Build history of the part. All positions in model axes, mm. Face numbers are marked on the shaded views. Round coordinates to 2 decimals unless told otherwise and drop trailing zeros. Order: outer loops, then holes, each group sorted by start corner. A loop starts at its lowest first (then second) coordinate and runs counter-clockwise, first axis right, second up. Notation, with made-up numbers: M -19.75,-11.75 L 19.25,-11.75 A13 cw 19.25,-7.75 Z; hole C -21.75,17.25 d4. An arc over 180 degrees is marked long. Use CSV: the item, a comma, the result in double quotes.
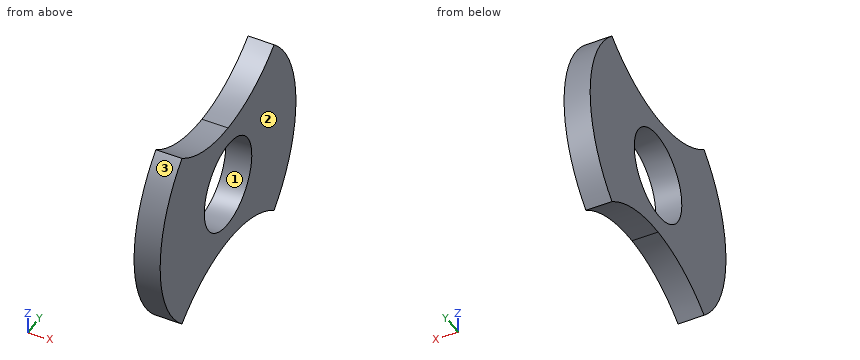
from build123d import *

# Parameters (mm, degrees)
BOSS_EXTRUDE1_DEPTH = 10
SKETCH3_R           = 17.5
CUT_EXTRUDE3_DEPTH  = 63.842489918


with BuildPart() as part:
    # Sketch1 → Boss-Extrude1 (new body)
    with BuildSketch(Plane(origin=(0, 0, 0), x_dir=(0, 0, -1), z_dir=(1, 0, 0))):
        with BuildLine():
            ThreePointArc((-36.722656494, 33.942179351), (-28.013204115, 17.954750168), (-25, 0))
            ThreePointArc((-25, 0), (-28.013204115, -17.954750168), (-36.722656494, -33.942179351))
            ThreePointArc((-36.722656494, -33.942179351), (0, -50.00625), (36.722656494, -33.942179351))
            ThreePointArc((36.722656494, -33.942179351), (28.013204115, -17.954750168), (25, 0))
            ThreePointArc((25, 0), (28.013204115, 17.954750168), (36.722656494, 33.942179351))
            ThreePointArc((36.722656494, 33.942179351), (0, 50.00625), (-36.722656494, 33.942179351))
        make_face()
    extrude(amount=BOSS_EXTRUDE1_DEPTH)

    # Sketch3 → Cut-Extrude3 (cut, through all)
    with BuildSketch(Plane(origin=(0, 0, 0), x_dir=(0, 0, -1), z_dir=(1, 0, 0))):
        Circle(SKETCH3_R)
    extrude(amount=CUT_EXTRUDE3_DEPTH, mode=Mode.SUBTRACT)


solid = part.part
(1) Wall check: line 1 (Y direction, x = 5.25, z = 0); line 2 (Z direction, x = 1.25, y = 7); line 3 (Z direction, x = 8.5, y = -13). Give the ranges that are in metal, low to high. Write a range as from..to.
Answer block:
line 1,"y = -50.01..-17.5, 17.5..50.01"
line 2,"z = -25.45..-16.04, 16.04..25.45"
line 3,"z = -26.56..-11.72, 11.72..26.56"
(2) Drop flat-ended pins along their axis: pin 1 (1.5 mm diameter, centred on x = 7, z = -13.5, fed in from +Y); pin 2 (1.5 mm diameter, centred on x = 2, z = 22.5, fed in from +Y); pin 3 (3 mm diameter, centred on x = 3, z = -28.5, fed in from -Y). Give the stop position or say it passes through.
Answer block:
pin 1,"stops at y = 48.35"
pin 2,"stops at y = 45.03"
pin 3,"stops at y = -42.09"
(3) Cut at C-C, the plane y = 11.5. Give the cut face in (x, z), and give its area (3 significant figures).
Answer block:
outline,"M 0,-26.22 L 10,-26.22 L 10,-13.19 L 0,-13.19 Z; M 0,13.19 L 10,13.19 L 10,26.22 L 0,26.22 Z"
area,"260 mm²"
(4) Cut at B-B, the plane z = 0. Give the cut face in (x, y), and give its area (3 significant figures).
Answer block:
outline,"M 0,-50.01 L 10,-50.01 L 10,-17.5 L 0,-17.5 Z; M 0,17.5 L 10,17.5 L 10,50.01 L 0,50.01 Z"
area,"650 mm²"
(5) Two-plate mould, pull along Y, no slides. Class the marked faces 1, 2 and 3: released by +Y, released by -Y, zero draft, split by the parting line, or undercut.
Answer block:
face 1,"undercut"
face 2,"zero draft"
face 3,"released by -Y"
(6) Cut at A-A, the plane x = 8.25. Give the cut face in (y, z).
Answer block:
outline,"M -33.94,-36.72 A55 cw 33.94,-36.72 A50.01 ccw 33.94,36.72 A55 cw -33.94,36.72 A50.01 ccw Z; hole C 0,0 d35"
(7) Cut at D-D, the plane y = -37.5. Give the cut face in (x, z).
Answer block:
outline,"M 0,-33.08 L 10,-33.08 L 10,33.08 L 0,33.08 Z"
